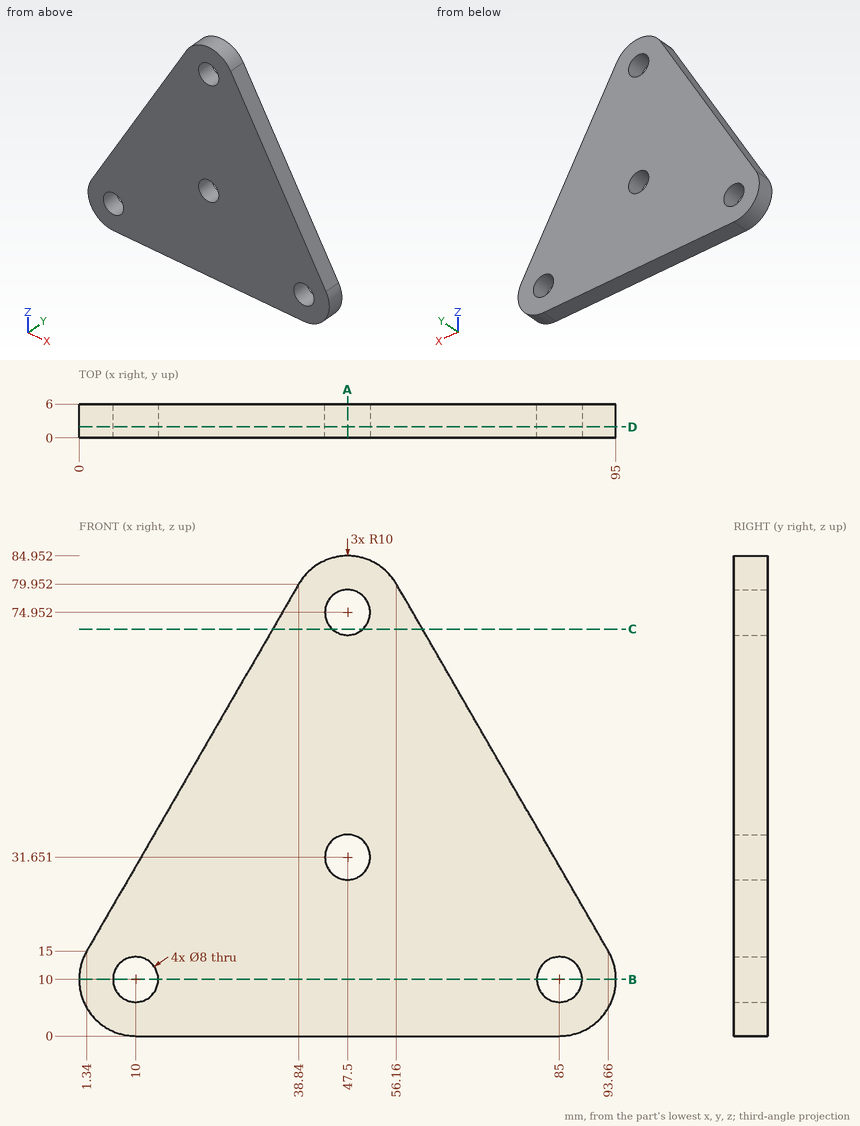
Geometry check sheet. Reference: drawing and pictorial views, mm from the part's lowest x, y, z. Give positions to 0.01 mm unless a question says otherwise; leave off trailing zeros. Loops run counter-clockwise (first coordinate to the right, second up) from the corner with the lowest first, then second, coordinate; pieces in that order, holes last.
1. Section check A-A, the plane x = 47.5. Enter the section's corners in (y, z).
2. Section check B-B, the plane z = 10. Enter the section's corners in (x, y).
3. Section check C-C, the plane z = 72. Enter the section's corners in (x, y), then the cut area to 3 significant figures.
4. Thickness scan on line 1 (Z direction, x = 46.5, y = 2.65) (1 decimal); line 2 (X direction, y = 2.45, z = 15); line 3 (Z direction, x = 86.5, y = 1.25) (1 decimal). Record the ranges inside material, lowest first.
5. Go/stop test with a flat-tipped pin: pin 1 Ø6.5 at (x, z) = (10, 10) entering from +Y. Record where the tip stops, or that it passes through.
6. Section check D-D, the plane y = 1.95. Enter the section's corners in (x, z), then the cut area to 3 significant figures.
Geometry says:
1. outline: (0, 0) - (6, 0) - (6, 27.65) - (0, 27.65) - close; (0, 35.65) - (6, 35.65) - (6, 70.95) - (0, 70.95) - close; (0, 78.95) - (6, 78.95) - (6, 84.95) - (0, 84.95) - close
2. outline: (0, 0) - (6, 0) - (6, 6) - (0, 6) - close; (14, 0) - (81, 0) - (81, 6) - (14, 6) - close; (89, 0) - (95, 0) - (95, 6) - (89, 6) - close
3. outline: (34.25, 0) - (44.8, 0) - (44.8, 6) - (34.25, 6) - close; (50.2, 0) - (60.75, 0) - (60.75, 6) - (50.2, 6) - close
3. area: 127 mm2
4. line 1: z = 0 to 27.8, 35.5 to 71.1, 78.8 to 84.9
4. line 2: x = 1.34 to 93.66
4. line 3: z = 0.1 to 6.3, 13.7 to 27.4
5. pin 1: passes through
6. outline: (1.34, 15) arc R10 ccw to (10, 0) - (85, 0) arc R10 ccw to (93.66, 15) - (56.16, 79.95) arc R10 ccw to (38.84, 79.95) - close; hole circle Ø8 at (10, 10); hole circle Ø8 at (47.5, 31.65); hole circle Ø8 at (47.5, 74.95); hole circle Ø8 at (85, 10)
6. area: 4,800 mm2
